from build123d import *
from build123d.topology import SkipClean

# Parameters (mm, degrees)
SKETCH1_W           = 30
SKETCH1_H           = 30
SKETCH1_W_2         = 2
SKETCH1_H_2         = 10
BOSS_EXTRUDE1_DEPTH = 75
SKETCH2_W           = 30
SKETCH2_H           = 17.5
CUT_EXTRUDE1_DEPTH  = 75
SKETCH3_W           = 36
SKETCH3_H           = 30.162749864
CUT_EXTRUDE2_DEPTH  = 28
SKETCH5_R           = 2.5
CUT_EXTRUDE3_DEPTH  = 50
BOSS_EXTRUDE2_DEPTH = 2
BOSS_EXTRUDE3_START = 2
BOSS_EXTRUDE3_DEPTH = 2
SKETCH9_R           = 2.5
CUT_EXTRUDE4_DEPTH  = 169.967145294
SKETCH11_W          = 10
SKETCH11_H          = 40.338772632
SKETCH11_W_2        = 20
SKETCH11_H_2        = 5
BOSS_EXTRUDE4_DEPTH = 2
SKETCH13_W          = 25
SKETCH13_H          = 20
BOSS_EXTRUDE5_DEPTH = 2
SKETCH15_W          = 2
SKETCH15_H          = 20
BOSS_EXTRUDE6_DEPTH = 15
SKETCH16_W          = 80
SKETCH16_H          = 25
BOSS_EXTRUDE8_DEPTH = 2


with BuildPart() as part:
    # Sketch1 → Boss-Extrude1 (new body)
    with BuildSketch(Plane.XY):
        Rectangle(SKETCH1_W, SKETCH1_H)
        with BuildLine():
            Line((50.917737084, -85.641756384), (53, -85.641756384))
            ThreePointArc((53, -85.641756384), (42.989370072, -49.687860894), (15, -25))
            Line((15, -25), (14.157929479, -26.814088542))
            ThreePointArc((14.157929479, -26.814088542), (41.246515654, -50.786104008), (50.917737084, -85.641756384))
        make_face()
        with Locations((14, -20)):
            Rectangle(SKETCH1_W_2, SKETCH1_H_2)
        Polygon((14.157929479, -26.814088542), (15, -25), (13, -25), (13, -26.814088542), align=None)
        with BuildLine():
            Line((12.135037198, -143.180046466), (13, -144.983332176))
            ThreePointArc((13, -144.983332176), (41.796634815, -121.242036174), (53, -85.641756384))
            Line((53, -85.641756384), (50.917737084, -85.641756384))
            ThreePointArc((50.917737084, -85.641756384), (40.047121172, -120.154156399), (12.135037198, -143.180046466))
        make_face()
    extrude(amount=BOSS_EXTRUDE1_DEPTH)

    # Sketch2 → Cut-Extrude1 (cut)
    with BuildSketch(Plane(origin=(0, 15, 0), x_dir=(1, 0, 0), z_dir=(0, 1, 0))):
        with Locations((0, -8.75)):
            Rectangle(SKETCH2_W, SKETCH2_H)
        with Locations((0, -66.25)):
            Rectangle(SKETCH2_W, SKETCH2_H)
    extrude(amount=-CUT_EXTRUDE1_DEPTH, mode=Mode.SUBTRACT)

    # Sketch3 → Cut-Extrude2 (cut)
    with BuildSketch(Plane.ZY.offset(15)):
        with Locations((37.5, 0.030332794)):
            Rectangle(SKETCH3_W, SKETCH3_H)
    extrude(amount=-CUT_EXTRUDE2_DEPTH, mode=Mode.SUBTRACT)

    # Sketch5 → Cut-Extrude3 (cut)
    with BuildSketch(Plane.XY.offset(57.5)):
        Circle(SKETCH5_R)
    extrude(amount=-CUT_EXTRUDE3_DEPTH, mode=Mode.SUBTRACT)

    # Sketch6 → Boss-Extrude2 (add)
    with SkipClean():  # the faces are left unmerged after this step: merging them gives an invalid solid
        with BuildSketch(Plane.XY.offset(75)):
            with BuildLine():
                Line((13, -144.983332176), (13, -94.983332176))
                Line((13, -94.983332176), (52.174379027, -94.983332176))
                ThreePointArc((52.174379027, -94.983332176), (39.036739849, -125.036474764), (13, -144.983332176))
            make_face()
        extrude(amount=BOSS_EXTRUDE2_DEPTH)

    # Sketch7 → Boss-Extrude3 (add)
    with SkipClean():  # the faces are left unmerged after this step: merging them gives an invalid solid
        with BuildSketch(Plane(origin=(0, 0, 0), x_dir=(-1, 0, 0), z_dir=(0, 0, -1)).offset(BOSS_EXTRUDE3_START)):
            with BuildLine():
                Line((-13, -144.983332176), (-13, -94.983332176))
                Line((-13, -94.983332176), (-52.174379027, -94.983332176))
                ThreePointArc((-52.174379027, -94.983332176), (-39.036739849, -125.036474764), (-13, -144.983332176))
            make_face()
        extrude(amount=-BOSS_EXTRUDE3_DEPTH)

    # Sketch9 → Cut-Extrude4 (cut, through all)
    with SkipClean():  # the faces are left unmerged after this step: merging them gives an invalid solid
        with BuildSketch(Plane.ZY.offset(-13)):
            with Locations((35, -61.814088542)):
                Circle(SKETCH9_R)
        extrude(amount=-CUT_EXTRUDE4_DEPTH, mode=Mode.SUBTRACT)

    # Sketch11 → Boss-Extrude4 (add)
    with SkipClean():  # the faces are left unmerged after this step: merging them gives an invalid solid
        with BuildSketch(Plane(origin=(15, 0, 0), x_dir=(0, 0, -1), z_dir=(1, 0, 0))):
            with Locations((-42.5, -4.830613684)):
                Rectangle(SKETCH11_W, SKETCH11_H)
            with Locations((-32.5, -4.830613684)):
                Rectangle(SKETCH11_W, SKETCH11_H)
            with Locations((-37.5, 17.838772632)):
                Rectangle(SKETCH11_W_2, SKETCH11_H_2)
        extrude(amount=BOSS_EXTRUDE4_DEPTH)

    # Sketch13 → Boss-Extrude5 (add)
    with SkipClean():  # the faces are left unmerged after this step: merging them gives an invalid solid
        with BuildSketch(Plane(origin=(0, 20.338772632, 0), x_dir=(1, 0, 0), z_dir=(0, 1, 0))):
            with Locations((4.5, -37.5)):
                Rectangle(SKETCH13_W, SKETCH13_H)
        extrude(amount=BOSS_EXTRUDE5_DEPTH)

    # Sketch15 → Boss-Extrude6 (add)
    with SkipClean():  # the faces are left unmerged after this step: merging them gives an invalid solid
        with BuildSketch(Plane(origin=(0, 22.338772632, 0), x_dir=(1, 0, 0), z_dir=(0, 1, 0))):
            with Locations((-7, -37.5)):
                Rectangle(SKETCH15_W, SKETCH15_H)
        extrude(amount=BOSS_EXTRUDE6_DEPTH)

    # Sketch16 → Boss-Extrude8 (add)
    with SkipClean():  # the faces are left unmerged after this step: merging them gives an invalid solid
        with BuildSketch(Plane(origin=(0, 37.338772632, 0), x_dir=(1, 0, 0), z_dir=(0, 1, 0))):
            with Locations((-96, -50)):
                Rectangle(SKETCH16_W, SKETCH16_H)
            with Locations((-96, -25)):
                Rectangle(SKETCH16_W, SKETCH16_H)
            Polygon((-6, -77.5), (-6, -37.5), (-56, -37.5), (-56, -62.5), (-56, -77.5), align=None)
            Polygon((-56, -37.5), (-6, -37.5), (-6, 2.5), (-56, 2.5), (-56, -12.5), align=None)
        extrude(amount=BOSS_EXTRUDE8_DEPTH)


solid = part.part
Part model, mm, in its own coordinate system. A direction names the side the tool comes from. Coordinates: 2 decimals unless noted, no trailing zeros. Write each loop counter-clockwise with the first axis right and the second up, starting at its lowest first coordinate (ties: lowest second). Pieces come first, ordered by that corner, then holes. Notation, with made-up numbers: M -6,-28 L 41,-28 A21 ccw 41,-10 Z; hole C 56,79.25 d1. An arc over 180 degrees is marked long. Return JSON: item names as keys, results as strings.
1. 3-axis set-ups, long thin cutter, end or side, ignore diameter. For faces 1 (the face through (44, -55, 0)), 2 (the face through (13.3, 15, 37.4)), 3 (the face through (28, -113, 0)), 4 (the face through (16, 11, 47.5)): which of +Z, -Z, +X, -X, +Y, -Y reach the whole face in a straight line?
Determined:
{"face 1": "-Z, +X, -X, +Y", "face 2": "+Z, -Z, -X", "face 3": "-X", "face 4": "+Z, +X"}
2. Probe L1, parallel to Z at x = 26, y = -95.5; L2, parallel to Y at x = 0, z = 18.7; L3, parallel to Z at x = 12.5, y = -12. List the from-to ranges inside material, lowest first.
Determined:
{"L1": "-2 to 0, 75 to 77", "L2": "-15 to -2.5, 2.5 to 15", "L3": "17.5 to 19.5, 55.5 to 57.5"}
3. Saw through at A-A, the plane z = 9. Write the cut outline in (x, y).
Determined:
{"outline": "M -56,37.34 L -6,37.34 L -6,39.34 L -56,39.34 Z; M 12.14,-143.18 L 13,-144.98 A65.65 ccw 15,-25 L 15,-27.21 A63.71 cw Z"}
4. Pull direction Y, two halves, no side cores. Call faces 5 (the face through (28, -113, 75)), 6 (the face through (-0.54, -2.44, 56.51)), 7 (the face through (3, -1, 57.5)): pulls with the +Y half, pulls with the -Y half, needs draft (parallel to the pull), parting line crosses it, or undercut.
Determined:
{"face 5": "undercut", "face 6": "undercut", "face 7": "needs draft"}
5. Saw through at D-D, the plane z = 53. Write the cut outline in (x, y).
Determined:
{"outline": "M -136,37.34 L -6,37.34 L -6,39.34 L -136,39.34 Z; M 12.14,-143.18 L 13,-144.98 A65.65 ccw 15,-25 L 15,15 L 13,15 L 13,-26.81 L 14.16,-26.81 A63.71 cw Z"}
6. Saw through at C-C, the plane x = 0. Write the cut outline in (y, z), then the cut area to 3 significant figures.
Determined:
{"outline": "M -15,17.5 L -2.5,17.5 L -2.5,19.5 L -15,19.5 Z; M -15,55.5 L -2.5,55.5 L -2.5,57.5 L -15,57.5 Z; M 2.5,17.5 L 15,17.5 L 15,19.5 L 2.5,19.5 Z; M 2.5,55.5 L 15,55.5 L 15,57.5 L 2.5,57.5 Z; M 20.34,27.5 L 22.34,27.5 L 22.34,47.5 L 20.34,47.5 Z", "area": "140 mm²"}
7. Saw through at B-B, the plane y = 0. Write the cut outline in (x, z), then the cut area to 3 significant figures.
Determined:
{"outline": "M -15,17.5 L -2.5,17.5 L -2.5,19.5 L -15,19.5 Z; M -15,55.5 L -2.5,55.5 L -2.5,57.5 L -15,57.5 Z; M 2.5,17.5 L 15,17.5 L 15,27.5 L 17,27.5 L 17,47.5 L 15,47.5 L 15,57.5 L 2.5,57.5 L 2.5,55.5 L 13,55.5 L 13,19.5 L 2.5,19.5 Z", "area": "212 mm²"}
8. Flat gauge pins, fed straight in: pin 1 Ø8 at (y, z) = (17, 28) entering from +X; pin 2 Ø1.1 at (y, z) = (-26.5, 11.5) entering from -X; pin 3 Ø12 at (x, z) = (-10.5, 58.5) entering from -Y. Where does each tip first touch, or does it go through?
Determined:
{"pin 1": "x = 17", "pin 2": "x = 15", "pin 3": "y = -15"}
